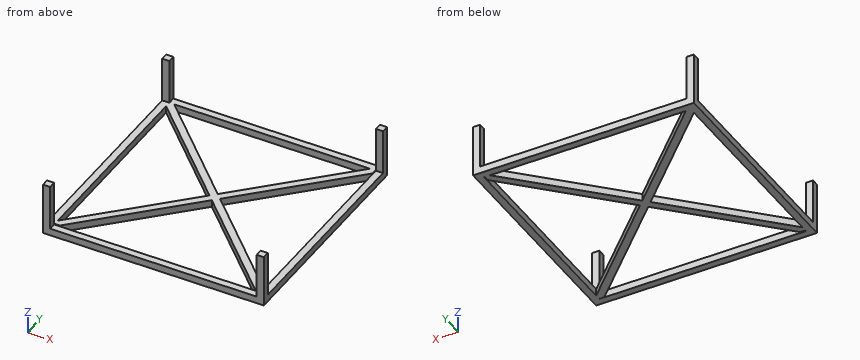
```python
from build123d import *

# Parameters (mm, degrees)
F0_W     = 30
F0_H     = 30
F0_W_2   = 870
F0_H_2   = 870
F2_DEPTH = 30
F3_DEPTH = 30
F4_W     = 30
F4_H     = 30
F5_DEPTH = 190
F6_DEPTH = 15


with BuildPart() as f2:
    # F0 (on Top) → F2 (new body)
    with BuildSketch(Plane.XY):
        with Locations((-435.5585327744, 814.4162455201)):
            Rectangle(F0_W, F0_H)
        with Locations((14.4414672256, 814.4162455201)):
            Rectangle(F0_W_2, F0_H)
        with Locations((-435.5585327744, 364.4162455201)):
            Rectangle(F0_W, F0_H_2)
        with Locations((464.4414672256, 814.4162455201)):
            Rectangle(F0_W, F0_H)
        with Locations((-435.5585327744, -85.5837544799)):
            Rectangle(F0_W, F0_H)
        with Locations((464.4414672256, 364.4162455201)):
            Rectangle(F0_W, F0_H_2)
        with Locations((14.4414672256, -85.5837544799)):
            Rectangle(F0_W_2, F0_H)
        with Locations((464.4414672256, -85.5837544799)):
            Rectangle(F0_W, F0_H)
    extrude(amount=-F2_DEPTH)

    # F1 (on face) → F3 (join)
    with BuildSketch(Plane.XY):
        Polygon((-420.9787249565, -43.7369011343), (-420.9787249565, -65.8913552761), (-398.8242447376, -65.8913552761), (12.1761524069, 344.280398684), (-10.0305031789, 366.3827953016), align=None)
        Polygon((12.2952993787, 388.6635861224), (-10.0305031789, 366.3827953016), (12.1761524069, 344.280398684), (34.4943990212, 366.5536481084), align=None)
        Polygon((-422.4041998386, 776.8204212189), (-10.0305031789, 366.3827953016), (12.2952993787, 388.6635861224), (-399.9607563019, 799.2638349533), align=None)
        Polygon((34.4943990212, 366.5536481084), (12.1761524069, 344.280398684), (427.7071654797, -69.2997202277), (449.8616158962, -47.1452660859), align=None)
        Polygon((-422.4041998386, 799.2638349533), (-422.4041998386, 776.8204212189), (-399.9607563019, 799.2638349533), align=None)
        Polygon((424.2987632751, 799.836397171), (12.2952993787, 388.6635861224), (34.4943990212, 366.5536481084), (446.4532732964, 777.6819467545), align=None)
        Polygon((449.8616158962, -47.1452660859), (427.7071654797, -69.2997202277), (449.8616158962, -69.2997202277), align=None)
        Polygon((446.4532732964, 799.836397171), (424.2987632751, 799.836397171), (446.4532732964, 777.6819467545), align=None)
    extrude(amount=-F3_DEPTH)

    # F4 (on face) → F5 (join)
    with BuildSketch(Plane.XY):
        with Locations((464.4414672256, 814.4162455201)):
            Rectangle(F4_W, F4_H)
        with Locations((-435.5585327744, -85.5837544799)):
            Rectangle(F4_W, F4_H)
        with Locations((464.4414672256, -85.5837544799)):
            Rectangle(F4_W, F4_H)
        with Locations((-435.5585327744, 814.4162455201)):
            Rectangle(F4_W, F4_H)
    extrude(amount=F5_DEPTH)

    # F1 (on face) → F6 (join)
    with BuildSketch(Plane.XY):
        Polygon((-420.9787249565, -43.7369011343), (-420.9787249565, -65.8913552761), (-398.8242447376, -65.8913552761), (12.1761524069, 344.280398684), (-10.0305031789, 366.3827953016), align=None)
        Polygon((12.2952993787, 388.6635861224), (-10.0305031789, 366.3827953016), (12.1761524069, 344.280398684), (34.4943990212, 366.5536481084), align=None)
        Polygon((-422.4041998386, 776.8204212189), (-10.0305031789, 366.3827953016), (12.2952993787, 388.6635861224), (-399.9607563019, 799.2638349533), align=None)
        Polygon((34.4943990212, 366.5536481084), (12.1761524069, 344.280398684), (427.7071654797, -69.2997202277), (449.8616158962, -47.1452660859), align=None)
        Polygon((-422.4041998386, 799.2638349533), (-422.4041998386, 776.8204212189), (-399.9607563019, 799.2638349533), align=None)
        Polygon((424.2987632751, 799.836397171), (12.2952993787, 388.6635861224), (34.4943990212, 366.5536481084), (446.4532732964, 777.6819467545), align=None)
        Polygon((449.8616158962, -47.1452660859), (427.7071654797, -69.2997202277), (449.8616158962, -69.2997202277), align=None)
        Polygon((446.4532732964, 799.836397171), (424.2987632751, 799.836397171), (446.4532732964, 777.6819467545), align=None)
    extrude(amount=-F6_DEPTH)


solid = f2.part
```
Work out the finished part from the listing and answer in its coordinate system (mm). Coordinates: 2 decimals unless noted, no trailing zeros. Loops run counter-clockwise (first coordinate to the right, second up) from the corner with the lowest first, then second, coordinate; pieces in that order, holes last. Notation, with made-up numbers: (-18.75, -3.5) - (17.25, -3.5) arc R30 cw to (17.25, 32.5) - close; hole circle Ø4 at (-24.5, 21). An arc over 180 degrees is marked (long way). Use a Markdown table: item, result.
Item 1: Consider probe 1 along X at (y, z) = (670.5, -2); probe 2 along Y at (x, z) = (-342.5, -15); probe 3 along X at (y, z) = (733, -16.5). Determine where each line is inside the solid, lowest interval first. Write a range as from..to.
Evaluation:
| item | result |
|---|---|
| probe 1 | x = -450.56..-420.56, -315.58..-270.68, 294.7..339.05, 449.44..479.44 |
| probe 2 | y = -100.58..-70.58, -9.68..34.58, 697.29..742.03, 799.42..829.42 |
| probe 3 | x = -450.56..-420.56, -378.38..-333.43, 357.33..401.68, 449.44..479.44 |
Item 2: Find section B-B, the plane y = 91. Determine the outline of the cut face in (x, z), and give its area (3 significant figures).
Evaluation:
| item | result |
|---|---|
| outline | (-450.56, -30) - (-420.56, -30) - (-420.56, 0) - (-450.56, 0) - close; (-285.97, -30) - (-241.62, -30) - (-241.62, 0) - (-285.97, 0) - close; (266.65, -30) - (311.16, -30) - (311.16, 0) - (266.65, 0) - close; (449.44, -30) - (479.44, -30) - (479.44, 0) - (449.44, 0) - close |
| area | 4,470 mm2 |
Item 3: Find section A-A, the plane z = 114. Determine the outline of the cut face in (x, y), and give its area (3 significant figures).
Evaluation:
| item | result |
|---|---|
| outline | (-450.56, -100.58) - (-420.56, -100.58) - (-420.56, -70.58) - (-450.56, -70.58) - close; (-450.56, 799.42) - (-420.56, 799.42) - (-420.56, 829.42) - (-450.56, 829.42) - close; (449.44, -100.58) - (479.44, -100.58) - (479.44, -70.58) - (449.44, -70.58) - close; (449.44, 799.42) - (479.44, 799.42) - (479.44, 829.42) - (449.44, 829.42) - close |
| area | 3,600 mm2 |
Item 4: Given pin 1 Ø24 at (x, y) = (-160.5, -82) entering from +Z, flat-ended and moving along its own axis, determine where the tip first touches the part or whether it passes through.
Evaluation:
| item | result |
|---|---|
| pin 1 | stops at z = 0 |
